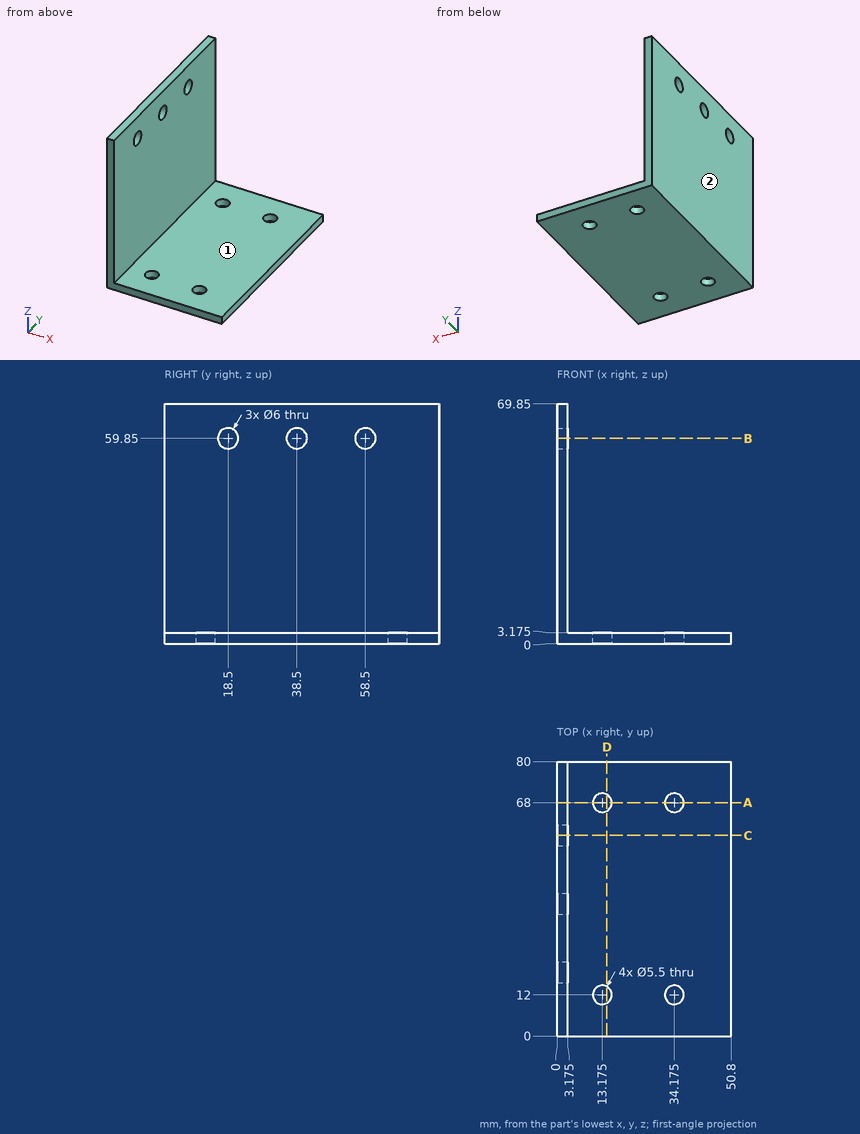
Answer from the drawing. Dimensions are ordinates in mm from the lowest x, y and z of the part. A direction names the side the tool comes from. Coordinates: 2 decimals unless noted, no trailing zeros. Loops run counter-clockwise (first coordinate to the right, second up) from the corner with the lowest first, then second, coordinate; pieces in that order, holes last.
Q1. Which of the six approach directions +Z, -Z, +X, -X, +Y, -Y give full straight-line access (tool end or side, diameter ignored) to the marked faces 1 and 2?
Q2. The part is cut by section A-A on y = 68. Write down the section's boundary in (x, z) (3 decimals).
Q3. The part is cut by section C-C on y = 58.5. Write down the section's boundary in (x, z) (3 decimals).
Q4. Each of these flat-tipped pins is pushed along its axis until it touches: pin 1 Ø3.5 at (x, y) = (13.175, 68) entering from -Z; pin 2 Ø6.5 at (x, y) = (34.175, 68) entering from +Z (3 decimals); pin 3 Ø8 at (y, z) = (55, 51.5) entering from +X (3 decimals). Where does it stop, or does it pass through?
Q5. The part is cut by section B-B on z = 59.85. Write down the section's boundary in (x, y) (3 decimals).
Q6. Consider probe 1 along Z at (x, y) = (2.25, 18.5); probe 2 along X at (y, z) = (58, 17) (3 decimals). Determine where each line is inside the solid, lowest interval first.
Q7. The part is cut by section D-D on x = 14.5. Write down the section's boundary in (y, z) (3 decimals).
Results below:
1. face 1: +Z, +X, +Y, -Y
1. face 2: +Z, -Z, -X, +Y, -Y
2. outline: (0, 0) - (10.425, 0) - (10.425, 3.175) - (3.175, 3.175) - (3.175, 69.85) - (0, 69.85) - close; (15.925, 0) - (31.425, 0) - (31.425, 3.175) - (15.925, 3.175) - close; (36.925, 0) - (50.8, 0) - (50.8, 3.175) - (36.925, 3.175) - close
3. outline: (0, 0) - (50.8, 0) - (50.8, 3.175) - (3.175, 3.175) - (3.175, 56.85) - (0, 56.85) - close; (0, 62.85) - (3.175, 62.85) - (3.175, 69.85) - (0, 69.85) - close
4. pin 1: passes through
4. pin 2: stops at z = 3.175
4. pin 3: stops at x = 3.175
5. outline: (0, 0) - (3.175, 0) - (3.175, 15.5) - (0, 15.5) - close; (0, 21.5) - (3.175, 21.5) - (3.175, 35.5) - (0, 35.5) - close; (0, 41.5) - (3.175, 41.5) - (3.175, 55.5) - (0, 55.5) - close; (0, 61.5) - (3.175, 61.5) - (3.175, 80) - (0, 80) - close
6. probe 1: z = 0 to 56.85, 62.85 to 69.85
6. probe 2: x = 0 to 3.175
7. outline: (0, 0) - (9.59, 0) - (9.59, 3.175) - (0, 3.175) - close; (14.41, 0) - (65.59, 0) - (65.59, 3.175) - (14.41, 3.175) - close; (70.41, 0) - (80, 0) - (80, 3.175) - (70.41, 3.175) - close
